from build123d import *

# Parameters (mm, degrees)
SKETCH1_W                      = 89.225
SKETCH1_H                      = 307.5
SKETCH1_W_2                    = 69.225
SKETCH1_H_2                    = 42
SKETCH1_H_3                    = 20
SKETCH1_H_4                    = 51
SKETCH1_H_5                    = 14.3
SKETCH1_H_6                    = 25
BOSS_EXTRUDE1_DEPTH            = 2
SKETCH20_W                     = 22
SKETCH20_H                     = 1
BOSS_EXTRUDE7_DEPTH            = 2
SKETCH21_W                     = 22
SKETCH21_H                     = 2
BOSS_EXTRUDE8_DEPTH            = 12
FILLET7_R                      = 2
FILLET8_R                      = 1
M2_5_CLEARANCE_HOLE3_D         = 2.9
SKETCH28_W                     = 12
SKETCH28_H                     = 1
BOSS_EXTRUDE11_DEPTH           = 2
SKETCH29_W                     = 12
SKETCH29_H                     = 2
BOSS_EXTRUDE12_DEPTH           = 12
FILLET11_R                     = 2
FILLET12_R                     = 1
M2_5_START                     = -286.2
M2_5_CLEARANCE_HOLE5_OUTLINE_R = 1.45
M2_5_CLEARANCE_HOLE5_DEPTH     = 80
M2_5_CLEARANCE_HOLE6_D         = 2.9
M2_CLEARANCE_HOLE1_D           = 2.4
M2_CLEARANCE_HOLE3_D           = 2.4


# Read off the part's stored shape, not the designer's step: M2.5 Clearance Hole5
with BuildPart() as part:
    # Sketch1 → Boss-Extrude1 (new body)
    with BuildSketch(Plane(origin=(0, 0, 0), x_dir=(1, 0, 0), z_dir=(0, 1, 0))):
        with Locations((44.6125, 153.75)):
            Rectangle(SKETCH1_W, SKETCH1_H)
        with Locations((44.6125, 246.2)):
            Rectangle(SKETCH1_W_2, SKETCH1_H_2, mode=Mode.SUBTRACT)
        Polygon((10, 16), (79.225, 16), (79.225, 21.8), (79.225, 27.8), (79.225, 39.6), (56.6125, 39.6), (32.6125, 39.6), (10, 39.6), (10, 27.8), align=None, mode=Mode.SUBTRACT)
        Polygon((10, 45.6), (79.225, 45.6), (79.225, 57.4), (56.6125, 57.4), (32.6125, 57.4), (10, 57.4), align=None, mode=Mode.SUBTRACT)
        Polygon((10, 63.4), (79.225, 63.4), (79.225, 75.2), (56.6125, 75.2), (32.6125, 75.2), (10, 75.2), align=None, mode=Mode.SUBTRACT)
        with Locations((44.6125, 91.2)):
            Rectangle(SKETCH1_W_2, SKETCH1_H_3, mode=Mode.SUBTRACT)
        with Locations((44.6125, 142.7)):
            Rectangle(SKETCH1_W_2, SKETCH1_H_4, mode=Mode.SUBTRACT)
        with Locations((44.6125, 290.35)):
            Rectangle(SKETCH1_W_2, SKETCH1_H_5, mode=Mode.SUBTRACT)
        with Locations((44.6125, 196.7)):
            Rectangle(SKETCH1_W_2, SKETCH1_H_6, mode=Mode.SUBTRACT)
    extrude(amount=BOSS_EXTRUDE1_DEPTH)

    # Sketch20 → Boss-Extrude7 (add)
    with BuildSketch(Plane(origin=(0, 0, 0), x_dir=(1, 0, 0), z_dir=(0, 1, 0))):
        with Locations((33.7, 184.7)):
            Rectangle(SKETCH20_W, SKETCH20_H)
    extrude(amount=BOSS_EXTRUDE7_DEPTH)

    # Sketch21 → Boss-Extrude8 (add)
    with BuildSketch(Plane(origin=(0, 0, 0), x_dir=(1, 0, 0), z_dir=(0, 1, 0))):
        with Locations((33.7, 186.2)):
            Rectangle(SKETCH21_W, SKETCH21_H)
    extrude(amount=BOSS_EXTRUDE8_DEPTH)

    # Fillet7
    fillet7_edges = [part.edges().sort_by_distance(p)[0] for p in [
        (33.7, 0, -187.2),
    ]]
    fillet(fillet7_edges, radius=FILLET7_R)

    # Fillet8
    fillet8_edges = [part.edges().sort_by_distance(p)[0] for p in [
        (33.7, 2, -185.2),
    ]]
    fillet(fillet8_edges, radius=FILLET8_R)

    # M2.5 Clearance Hole3 (through all)
    with Locations(Plane.XY.offset(-185.2)):
        with Locations((33.7, 7.4125)):
            Hole(M2_5_CLEARANCE_HOLE3_D / 2)

    # Sketch28 → Boss-Extrude11 (add)
    with BuildSketch(Plane(origin=(0, 0, 0), x_dir=(1, 0, 0), z_dir=(0, 1, 0))):
        with Locations((66.6125, 208.7)):
            Rectangle(SKETCH28_W, SKETCH28_H)
        with Locations((44.6125, 208.7)):
            Rectangle(SKETCH28_W, SKETCH28_H)
        with Locations((22.6125, 208.7)):
            Rectangle(SKETCH28_W, SKETCH28_H)
        with Locations((66.6125, 283.7)):
            Rectangle(SKETCH28_W, SKETCH28_H)
        with Locations((44.6125, 283.7)):
            Rectangle(SKETCH28_W, SKETCH28_H)
        with Locations((22.6125, 283.7)):
            Rectangle(SKETCH28_W, SKETCH28_H)
    extrude(amount=BOSS_EXTRUDE11_DEPTH)

    # Sketch29 → Boss-Extrude12 (add)
    with BuildSketch(Plane(origin=(0, 0, 0), x_dir=(1, 0, 0), z_dir=(0, 1, 0))):
        with Locations((66.6125, 207.2)):
            Rectangle(SKETCH29_W, SKETCH29_H)
        with Locations((44.6125, 207.2)):
            Rectangle(SKETCH29_W, SKETCH29_H)
        with Locations((22.6125, 207.2)):
            Rectangle(SKETCH29_W, SKETCH29_H)
        with Locations((66.6125, 285.2)):
            Rectangle(SKETCH29_W, SKETCH29_H)
        with Locations((44.6125, 285.2)):
            Rectangle(SKETCH29_W, SKETCH29_H)
        with Locations((22.6125, 285.2)):
            Rectangle(SKETCH29_W, SKETCH29_H)
    extrude(amount=BOSS_EXTRUDE12_DEPTH)

    # Fillet11
    fillet11_edges = [part.edges().sort_by_distance(p)[0] for p in [
        (66.6125, 0, -206.2),
        (44.6125, 0, -206.2),
        (22.6125, 0, -206.2),
        (66.6125, 0, -286.2),
        (44.6125, 0, -286.2),
        (22.6125, 0, -286.2),
    ]]
    fillet(fillet11_edges, radius=FILLET11_R)

    # Fillet12
    fillet12_edges = [part.edges().sort_by_distance(p)[0] for p in [
        (22.6125, 2, -284.2),
        (44.6125, 2, -284.2),
        (66.6125, 2, -284.2),
        (66.6125, 2, -208.2),
        (44.6125, 2, -208.2),
        (22.6125, 2, -208.2),
    ]]
    fillet(fillet12_edges, radius=FILLET12_R)

    # M2.5 Clearance Hole5 outline → M2.5 Clearance Hole5 (cut)
    with BuildSketch(Plane.XY.offset(M2_5_START)):
        with Locations((22.6125, 9.5)):
            Circle(M2_5_CLEARANCE_HOLE5_OUTLINE_R)
        with Locations((44.6125, 9.5)):
            Circle(M2_5_CLEARANCE_HOLE5_OUTLINE_R)
        with Locations((66.6125, 9.5)):
            Circle(M2_5_CLEARANCE_HOLE5_OUTLINE_R)
    extrude(amount=M2_5_CLEARANCE_HOLE5_DEPTH, mode=Mode.SUBTRACT)

    # M2.5 Clearance Hole6 (through all)
    with Locations(Plane(origin=(0, 2, 0), x_dir=(1, 0, 0), z_dir=(0, 1, 0))):
        with Locations((85.025, 4), (4.2, 4), (4.2, 109.2), (4.2, 176.2), (4.2, 303.5), (85.025, 303.5), (85.025, 176.2), (85.025, 109.2)):
            Hole(M2_5_CLEARANCE_HOLE6_D / 2)

    # M2 Clearance Hole1 (through all)
    with Locations(Plane(origin=(0, 0, 0), x_dir=(-1, 0, 0), z_dir=(0, -1, 0))):
        with Locations((-44.6125, 24.8), (-44.6125, 42.9), (-44.6125, 60.4), (-44.6125, 78.2)):
            Hole(M2_CLEARANCE_HOLE1_D / 2)

    # M2 Clearance Hole3 (through all)
    with Locations(Plane(origin=(0, 0, 0), x_dir=(-1, 0, 0), z_dir=(0, -1, 0))):
        with Locations((-44.6125, 13)):
            Hole(M2_CLEARANCE_HOLE3_D / 2)


solid = part.part
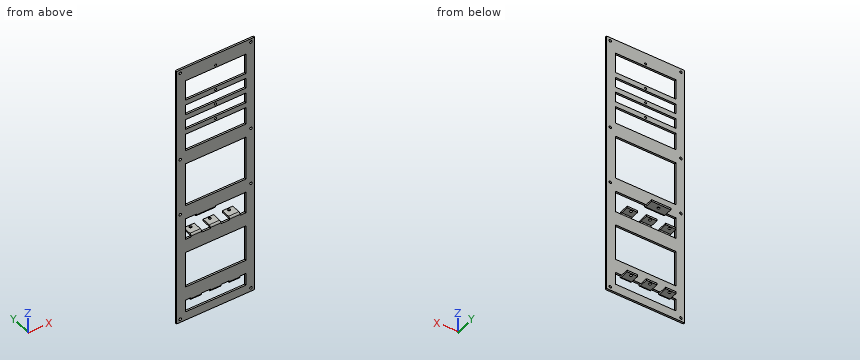
Read the model definition and answer for the solid it produces. Units are mm, in the model's axes. Give positions to 0.01 mm unless a question says otherwise; leave off trailing zeros. Write each loop counter-clockwise with the first axis right and the second up, starting at its lowest first coordinate (ties: lowest second). Pieces come first, ordered by that corner, then holes. Notation, with made-up numbers: (66, 15.5) - (105, 15.5) arc R29 ccw to (105, 44.5) - close; hole circle Ø5 at (-36.5, 51). An arc over 180 degrees is marked (long way). Answer in a Markdown table with one row per item. Add a question column.
Item 1: Find the intervals of material crossed by L1, parallel to X at y = 0.4, z = -176.2 (3 decimals); L2, parallel to Z at x = 68, y = 4; L3, parallel to Z at x = 23.5, y = 3.25, in increasing order.
Item 2: Section A-A, the plane z = -72.5 is taken. Write down the section's boundary in (x, y) (3 decimals), and give its area (3 significant figures).
Item 3: Flat-ended cylindrical pins translate along their axes: P1, Ø2.5, axis at x = 25.5, y = 6.5, coming from the -Z side; P2, Ø1.6, axis at x = 76, y = 0.5, coming from the +Z side; P3, Ø4, axis at x = 85.025, z = -109.2, coming from the +Y side; P4, Ø2.5, axis at y = 5.5, z = -284.5, coming from the +X side. Find the tip coordinate at first contact, or state that the pin passes through.
Recorded:
| question | item | result |
|---|---|---|
| 1 | L1 | x = 0 to 2.75, 5.65 to 83.575, 86.475 to 89.225 |
| 1 | L2 | z = -286.2 to -284.2, -208.2 to -206.2 |
| 1 | L3 | z = -286.2 to -284.2, -208.2 to -206.2, -187.2 to -185.2 |
| 2 | outline | (0, 0) - (10, 0) - (10, 2) - (0, 2) - close; (79.225, 0) - (89.225, 0) - (89.225, 2) - (79.225, 2) - close |
| 2 | area | 40.0 mm2 |
| 3 | P1 | stops at z = -286.2 |
| 3 | P2 | stops at z = 0 |
| 3 | P3 | stops at y = 2 |
| 3 | P4 | stops at x = 72.61 |
